Can you work these out from the drawing? Everything is in mm from the part's minimum corner. Give positions to 0.01 mm unless a question says otherwise; leave off trailing zeros. Loops run counter-clockwise (first coordinate to the right, second up) from the corner with the lowest first, then second, coordinate; pieces in that order, holes last.
Q1. If we section it at A-A (y = 2.5): Please give me the cut outline in (x, z).
Q2. I need wall thicknesses on line 1 (Y direction, x = 0.8, z = 3.25); line 2 (Y direction, x = 0.3, z = 2.75); line 3 (Y direction, x = 1.1, z = 4.25) (1 decimal). Which ranges of each line are inside material? Lowest first, please.
Q3. If we section it at C-C (y = 0.75): Please give me the cut outline in (x, z) (1 decimal).
Q4. If we section it at B-B (z = 3.25): Please give me the cut outline in (x, y), plus the area to 3 significant figures.
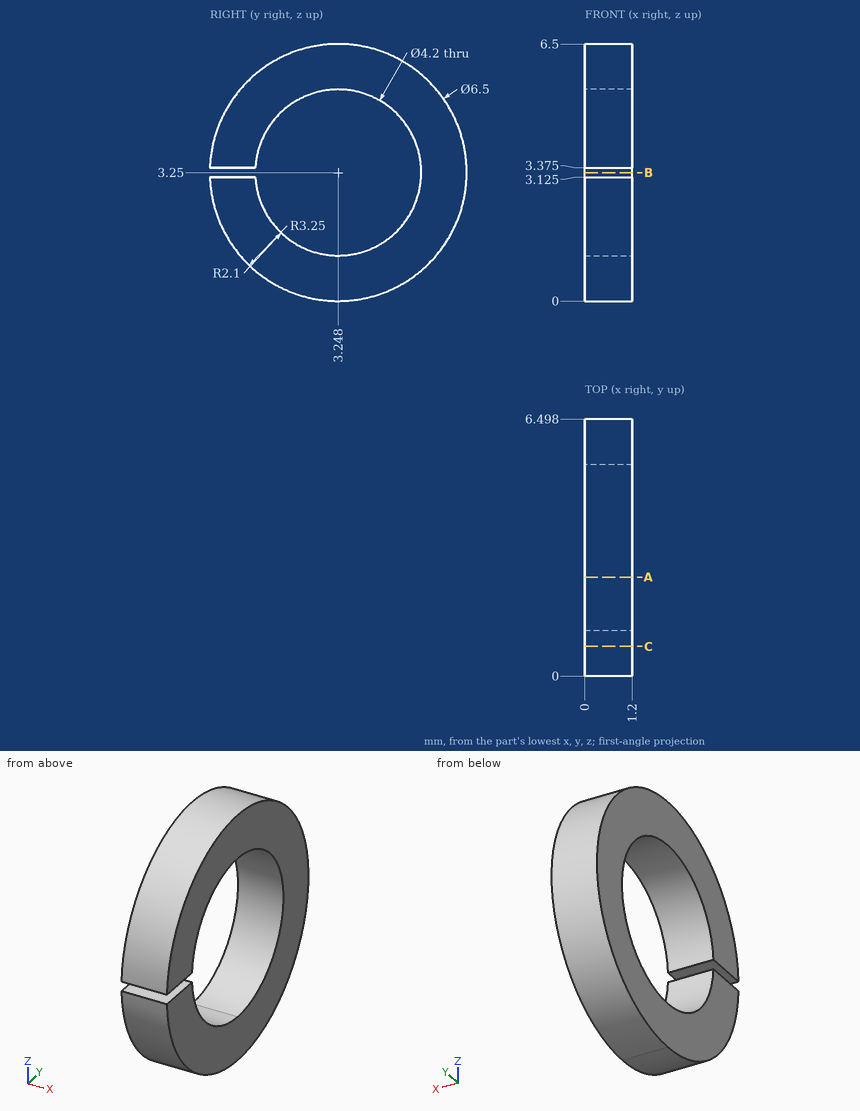
Check sheet entries:
1. outline: (0, 0.09) - (1.2, 0.09) - (1.2, 1.29) - (0, 1.29) - close; (0, 5.21) - (1.2, 5.21) - (1.2, 6.41) - (0, 6.41) - close
2. line 1: y = 5.35 to 6.5
2. line 2: y = 0.04 to 1.21, 5.29 to 6.46
2. line 3: y = 0.2 to 1.4, 5.1 to 6.3
3. outline: (0, 1.2) - (1.2, 1.2) - (1.2, 3.1) - (0, 3.1) - close; (0, 3.4) - (1.2, 3.4) - (1.2, 5.3) - (0, 5.3) - close
4. outline: (0, 5.35) - (1.2, 5.35) - (1.2, 6.5) - (0, 6.5) - close
4. area: 1.38 mm2
